Can you work these out from the drawing? Everything is in mm from the part's minimum corner. A direction names the side the tool comes from. Coordinates: 2 decimals unless noted, no trailing zeros. Order: outer loops, then holes, each group sorted by start corner. A loop starts at its lowest first (then second) coordinate and runs counter-clockwise, first axis right, second up. Notation, with made-up numbers: (0.25, -30) - (39.25, -30) arc R23 cw to (39.25, -16) - close; hole circle Ø5 at (29, 83.25). An arc over 180 degrees is marked (long way). Answer as CSV lines item,"result". Start each with the question number.
Item 1: I need wall thicknesses on line 1 (X direction, y = 2.5, z = 16); line 2 (Y direction, x = 6, z = 25.5) (3 decimals); line 3 (X direction, y = 6.35, z = 19.6). Which ranges of each line are inside material? Lowest first, please.
Item 2: Imagine slicing it at B-B on z = 13.5. List the corners of the cut face in (x, y) for me (1 decimal).
Item 3: I'm going to push flat-ended pins straight in: pin 1 (5 mm diameter, centred on y = 2, z = 4, fed in from -X); pin 2 (2 mm diameter, centred on x = 15.875, y = 6.35, fed in from -Z) (3 decimals); pin 3 (3.5 mm diameter, centred on x = 28.575, z = 15.875, fed in from +Y) (3 decimals). Where does each tip first touch, or does it pass through?
Item 4: Imagine slicing it at D-D on y = 2.25. Count the separate pieces of the cut face and the enclosed holes in it, and give its area (3 significant figures).
Item 5: On a 3-axis mill with a long thin cutter (end or side, diameter ignored), from which of +Z, -Z, +X, -X, +Y, -Y can I reach the whole of each face in a straight line? I mean the marked faces 4 and 5. Say none if no direction works.
Item 6: We'd pull the mould along X, two halves only. Please class the marked faces 1, 2 and 3: pulls with the +X half, pulls with the -X half, needs draft (parallel to the pull), parting line crosses it, or undercut.
Item 7: Imagine slicing it at A-A on x = 29.5. List the corners of the cut face in (y, z) for me (3 decimals), and give its area (3 significant figures).
Item 8: Imagine slicing it at C-C on x = 21.5. List the corners of the cut face in (y, z) for me (1 decimal).
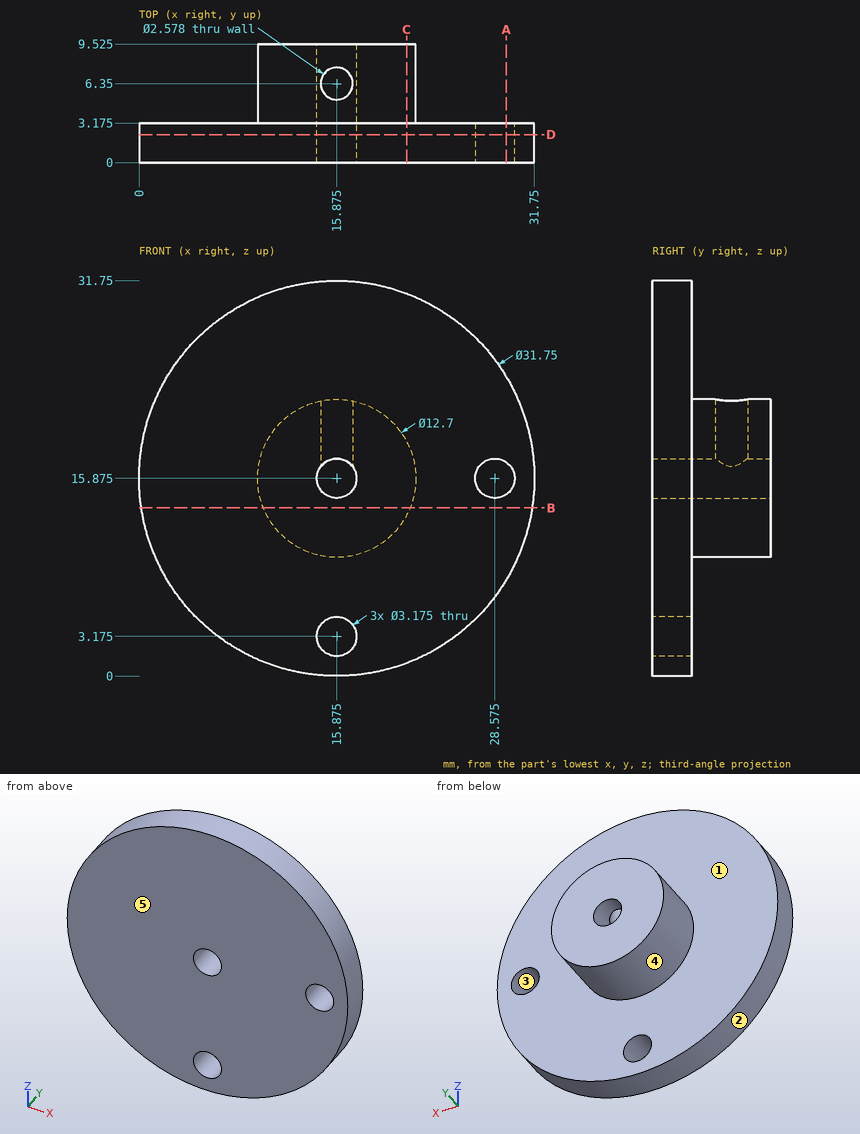
Responses:
1,line 1,"x = 0 to 14.29, 17.46 to 26.99, 30.16 to 31.75"
1,line 2,"y = 0 to 3.175"
1,line 3,"x = 10.73 to 14.59, 17.16 to 21.02"
2,outline,"(0.2, 0) - (31.6, 0) - (31.6, 3.2) - (21.8, 3.2) - (21.8, 9.5) - (10, 9.5) - (10, 3.2) - (0.2, 3.2) - close"
3,pin 1,"stops at x = 3.06"
3,pin 2,"stops at z = 9.525"
3,pin 3,"stops at y = 3.175"
4,separate pieces,"1"
4,enclosed holes,"3"
4,area,"768 mm^2"
5,face 4,"+Y"
5,face 5,"+Z, -Z, +X, -X, -Y"
6,face 1,"needs draft"
6,face 2,"parting line crosses it"
6,face 3,"undercut"
7,outline,"(0, 7.728) - (3.175, 7.728) - (3.175, 14.585) - (0, 14.585) - close; (0, 17.165) - (3.175, 17.165) - (3.175, 24.022) - (0, 24.022) - close"
7,area,"43.5 mm^2"
8,outline,"(0, 1) - (3.2, 1) - (3.2, 12.9) - (9.5, 12.9) - (9.5, 18.8) - (3.2, 18.8) - (3.2, 30.7) - (0, 30.7) - close"
